Read the model definition and answer for the solid it produces. Units are mm, in the model's axes. A direction names the side the tool comes from. Coordinates: 2 decimals unless noted, no trailing zeros. Write each loop counter-clockwise with the first axis right and the second up, starting at its lowest first coordinate (ties: lowest second). Pieces come first, ordered by that corner, then holes. Notation, with made-up numbers: (49, 89) - (57, 89) arc R17 ccw to (57, 113) - close; hole circle Ø4 at (11.5, 35.25). An arc over 180 degrees is marked (long way). Return JSON: item names as keys, results as strings.
```python
from build123d import *

# Parameters (mm, degrees)
F0_W     = 69.85
F0_H     = 44.45
F1_DEPTH = 3.175
F3_DEPTH = 3.175
F4_W     = 69.85
F4_H     = 44.45
F4_W_2   = 63.5
F4_H_2   = 38.1
F5_DEPTH = 38.1


with BuildPart() as f1:
    # F0 (on Top) → F1 (new body)
    with BuildSketch(Plane.XY):
        with Locations((34.925, -22.225)):
            Rectangle(F0_W, F0_H)
    extrude(amount=F1_DEPTH)

    # F2 (on face) → F3 (cut, through all)
    with BuildSketch(Plane.XY.offset(3.175)):
        with BuildLine():
            ThreePointArc((16.383, -22.225), (19.685, -25.527), (22.987, -22.225))
            Line((22.987, -22.225), (16.383, -22.225))
        make_face()
        with BuildLine():
            Line((16.383, -22.225), (22.987, -22.225))
            ThreePointArc((22.987, -22.225), (19.685, -18.923), (16.383, -22.225))
        make_face()
        with BuildLine():
            ThreePointArc((53.467, -22.225), (50.165, -18.923), (46.863, -22.225))
            Line((46.863, -22.225), (53.467, -22.225))
        make_face()
        with BuildLine():
            Line((53.467, -22.225), (46.863, -22.225))
            ThreePointArc((46.863, -22.225), (50.165, -25.527), (53.467, -22.225))
        make_face()
    extrude(amount=-F3_DEPTH, mode=Mode.SUBTRACT)

    # F4 (on face) → F5 (join)
    with BuildSketch(Plane.XY.offset(3.175)):
        with Locations((34.925, -22.225)):
            Rectangle(F4_W, F4_H)
        with Locations((34.925, -22.225)):
            Rectangle(F4_W_2, F4_H_2, mode=Mode.SUBTRACT)
    extrude(amount=F5_DEPTH)


solid = f1.part
```
(1) A cutting plane is placed at D-D (y = -5.5). Determine the outline of the cut face in (x, z) (3 decimals).
Answer:
{"outline": "(0, 0) - (69.85, 0) - (69.85, 41.275) - (66.675, 41.275) - (66.675, 3.175) - (3.175, 3.175) - (3.175, 41.275) - (0, 41.275) - close"}
(2) Determine the mould class of faces 1 (the face through (69.85, -23, 20)), 2 (the face through (0, -23, 20)), 3 (the face through (17.251, -19.993, 1.61)), 4 (the face through (34, -22, 0)) for opening direction X: +X half, -X half, draft (parallel to the pull), parting line (faces both ways), or undercut.
Answer:
{"face 1": "+X half", "face 2": "-X half", "face 3": "undercut", "face 4": "draft"}
(3) A flat-ended cylindrical pin translates along its axis: P1, Ø3, axis at x = 14.5, y = -17, coming from the +Z side (3 decimals). Find the tip coordinate at first contact, or state that the pin passes through.
Answer:
{"P1": "z = 3.175"}
(4) A cutting plane is placed at A-A (z = 17). Determine the outline of the cut face in (x, y) (3 decimals).
Answer:
{"outline": "(0, -44.45) - (69.85, -44.45) - (69.85, 0) - (0, 0) - close; hole (3.175, -41.275) - (66.675, -41.275) - (66.675, -3.175) - (3.175, -3.175) - close"}
(5) A cutting plane is placed at C-C (y = -24.5). Determine the outline of the cut face in (x, z) (3 decimals).
Answer:
{"outline": "(0, 0) - (17.292, 0) - (17.292, 3.175) - (3.175, 3.175) - (3.175, 41.275) - (0, 41.275) - close; (22.078, 0) - (47.772, 0) - (47.772, 3.175) - (22.078, 3.175) - close; (52.558, 0) - (69.85, 0) - (69.85, 41.275) - (66.675, 41.275) - (66.675, 3.175) - (52.558, 3.175) - close"}
(6) Straight lines are drawn through the part: line 1 (Y direction, x = 17.5, z = 33) (3 decimals); line 2 (X direction, y = -21.5, z = 10) (3 decimals); line 3 (Z direction, x = 54, y = -33) (3 decimals). For each, find the intervals that lie inside material, in ascending order. Write a range as from..to.
Answer:
{"line 1": "-44.45..-41.275, -3.175..0", "line 2": "0..3.175, 66.675..69.85", "line 3": "0..3.175"}
(7) Which of the six approach directions +Z, -Z, +X, -X, +Y, -Y give full straight-line access (tool end or side, diameter ignored) to faces 5 (the face through (66.675, -22, 22)), 6 (the face through (34, 0, 20))?
Answer:
{"face 5": "+Z", "face 6": "+Z, -Z, +X, -X, +Y"}
(8) A cutting plane is placed at B-B (x = 8.5). Determine the outline of the cut face in (y, z) (3 decimals).
Answer:
{"outline": "(-44.45, 0) - (0, 0) - (0, 41.275) - (-3.175, 41.275) - (-3.175, 3.175) - (-41.275, 3.175) - (-41.275, 41.275) - (-44.45, 41.275) - close"}
